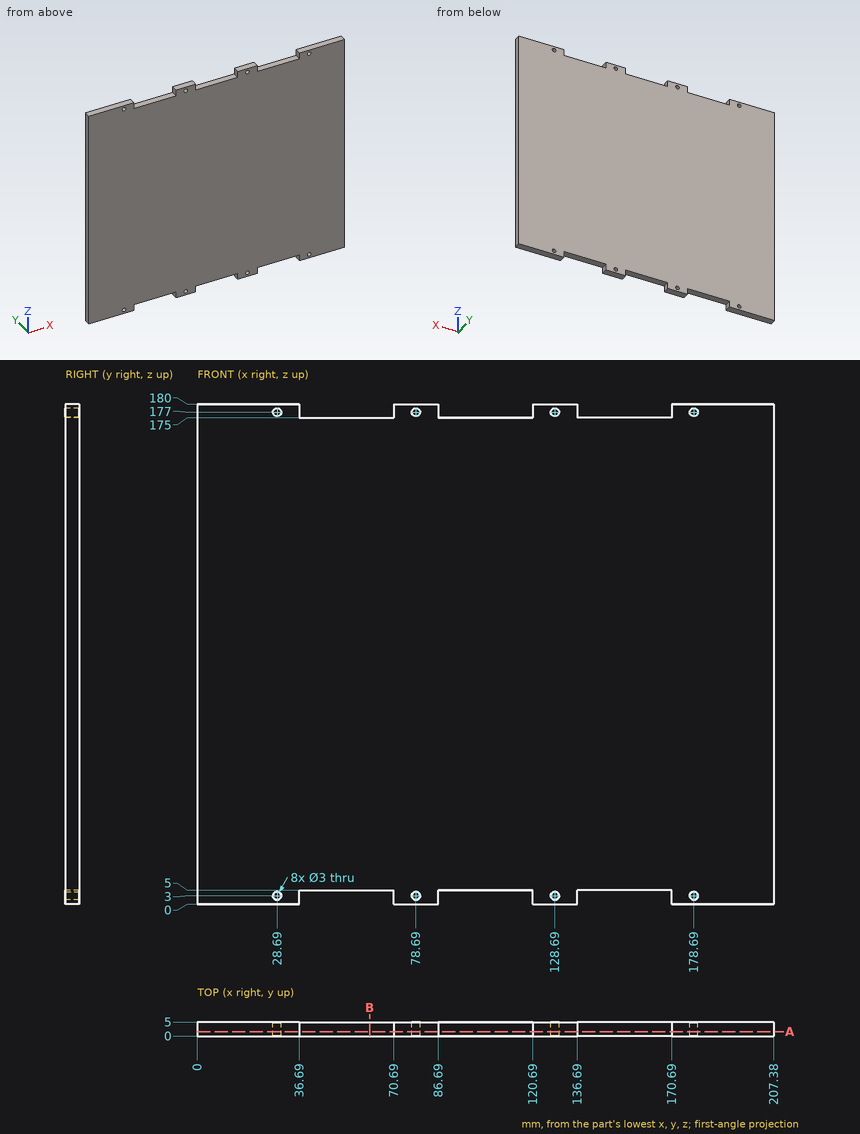
Answer from the drawing. Dimensions are ordinates in mm from the lowest x, y and z of the part. Give positions to 0.01 mm unless a question says otherwise; leave off trailing zeros. Order: outer loops, then holes, each group sorted by start corner. A loop starts at its lowest first (then second) coordinate and runs counter-clockwise, first axis right, second up. Notation, with made-up numbers: (6, 0) -> (14, 0) arc R22 ccw to (14, 18) -> close; hole circle Ø6 at (79, -7). An arc over 180 degrees is marked (long way). Answer as a JSON object with one key per item and string values. Group by question number.
1. Section B-B on x = 62 is taken. Determine the outline of the cut face in (y, z), plus the area to 3 significant figures.
2. Consider line 1 along Z through (x, y) = (28.69, 2.05); line 2 along Z through (x, y) = (106, 1.25). Determine where each line is inside the solid, lowest interval first. Write a range as [from, to].
3. A flat-ended cylindrical pin translates along its axis: pin 1 Ø1.5 at (x, y) = (105, 3.5) entering from -Z. Find the tip coordinate at first contact, or state that the pin passes through.
4. Section A-A on y = 1.55 is taken. Count the separate pieces of the cut face and the enclosed holes in it, plus the area to 3 significant figures.
Result sheet:
{
 "1": {"outline": "(0, 5) -> (5, 5) -> (5, 175) -> (0, 175) -> close", "area": "850 mm^2"},
 "2": {"line 1": "z = [0, 1.5], [4.5, 175.5], [178.5, 180]", "line 2": "z = [5, 175]"},
 "3": {"pin 1": "stops at z = 5"},
 "4": {"separate pieces": "1", "enclosed holes": "8", "area": "36,300 mm^2"}
}
